For this review, take the finished solid that the model builds, in its own axes (mm). A direction names the side the tool comes from. Round coordinates to 2 decimals unless told otherwise and drop trailing zeros. Write each loop counter-clockwise with the first axis right and the second up, starting at its lowest first coordinate (ties: lowest second). Pieces come first, ordered by that corner, then holes. Notation, with made-up numbers: (-24.5, 69) -> (-19.5, 69) arc R30 cw to (-19.5, 101) -> close; hole circle Ø3 at (1.5, 21). An arc over 180 degrees is marked (long way). Answer in a Markdown table with one row per item. Add a question column.
```python
from build123d import *

# Parameters (mm, degrees)
SKETCH1_W                 = 322.453
SKETCH1_H                 = 14.859
BOSS_EXTRUDE1_DEPTH       = 9.398
SKETCH2_W                 = 6.35
SKETCH2_H                 = 13.335
CUT_EXTRUDE1_DEPTH        = 323.762823192
F_5_CLEARANCE_HOLE1_D     = 3.556
F_5_CLEARANCE_HOLE1_DEPTH = 1.524
F_5_CLEARANCE_HOLE2_D     = 3.556
F_5_CLEARANCE_HOLE2_DEPTH = 14.859
F_5_CLEARANCE_HOLE3_D     = 3.556
FILLET1_R                 = 0.635


with BuildPart() as part:
    # Sketch1 → Boss-Extrude1 (new body)
    with BuildSketch(Plane(origin=(-4.699, 0, 0), x_dir=(0, -1, 0), z_dir=(-1, 0, 0))):
        with Locations((-161.2265, -5.9055)):
            Rectangle(SKETCH1_W, SKETCH1_H)
    extrude(amount=-BOSS_EXTRUDE1_DEPTH)

    # Sketch2 → Cut-Extrude1 (cut, through all)
    with BuildSketch(Plane.XZ):
        with Locations((0, -6.6675)):
            Rectangle(SKETCH2_W, SKETCH2_H)
    extrude(amount=-CUT_EXTRUDE1_DEPTH, mode=Mode.SUBTRACT)

    # #5 Clearance Hole1
    with Locations(Plane(origin=(4.699, 0, 0), x_dir=(0, 0, -1), z_dir=(1, 0, 0))):
        with Locations((8.5725, 307.9115), (8.5725, 317.6905), (8.5725, 298.1325), (8.5725, 288.3535), (8.5725, 278.5745), (8.5725, 268.7955), (8.5725, 259.0165), (8.5725, 249.2375), (8.5725, 239.4585), (8.5725, 229.6795), (8.5725, 219.9005), (8.5725, 210.1215), (8.5725, 200.3425), (8.5725, 190.5635), (8.5725, 180.7845), (8.5725, 171.0055), (8.5725, 161.2265), (8.5725, 151.4475), (8.5725, 141.6685), (8.5725, 131.8895), (8.5725, 122.1105), (8.5725, 112.3315), (8.5725, 102.5525), (8.5725, 92.7735), (8.5725, 82.9945), (8.5725, 73.2155), (8.5725, 63.4365), (8.5725, 53.6575), (8.5725, 43.8785), (8.5725, 34.0995), (8.5725, 24.3205), (8.5725, 14.5415), (8.5725, 4.7625)):
            Hole(F_5_CLEARANCE_HOLE1_D / 2, depth=F_5_CLEARANCE_HOLE1_DEPTH)

    # #5 Clearance Hole2
    with Locations(Plane.XY.offset(1.524)):
        with Locations((0, 307.9115), (0, 317.6905), (0, 298.1325), (0, 288.3535), (0, 278.5745), (0, 268.7955), (0, 259.0165), (0, 249.2375), (0, 239.4585), (0, 229.6795), (0, 219.9005), (0, 210.1215), (0, 200.3425), (0, 190.5635), (0, 180.7845), (0, 171.0055), (0, 161.2265), (0, 151.4475), (0, 141.6685), (0, 131.8895), (0, 122.1105), (0, 112.3315), (0, 102.5525), (0, 92.7735), (0, 82.9945), (0, 73.2155), (0, 63.4365), (0, 53.6575), (0, 43.8785), (0, 34.0995), (0, 24.3205), (0, 14.5415), (0, 4.7625)):
            Hole(F_5_CLEARANCE_HOLE2_D / 2, depth=F_5_CLEARANCE_HOLE2_DEPTH)

    # #5 Clearance Hole3 (through all)
    with Locations(Plane(origin=(-3.175, 0, 0), x_dir=(0, 0, -1), z_dir=(1, 0, 0))):
        with Locations((8.5725, 307.9115), (8.5725, 317.6905), (8.5725, 298.1325), (8.5725, 288.3535), (8.5725, 278.5745), (8.5725, 268.7955), (8.5725, 259.0165), (8.5725, 249.2375), (8.5725, 239.4585), (8.5725, 229.6795), (8.5725, 219.9005), (8.5725, 210.1215), (8.5725, 200.3425), (8.5725, 190.5635), (8.5725, 180.7845), (8.5725, 171.0055), (8.5725, 161.2265), (8.5725, 151.4475), (8.5725, 141.6685), (8.5725, 131.8895), (8.5725, 122.1105), (8.5725, 112.3315), (8.5725, 102.5525), (8.5725, 92.7735), (8.5725, 82.9945), (8.5725, 73.2155), (8.5725, 63.4365), (8.5725, 53.6575), (8.5725, 43.8785), (8.5725, 34.0995), (8.5725, 24.3205), (8.5725, 14.5415), (8.5725, 4.7625)):
            Hole(F_5_CLEARANCE_HOLE3_D / 2)

    # Fillet1
    fillet1_edges = [part.edges().sort_by_distance(p)[0] for p in [
        (-3.937, 322.453, -13.335),
        (-3.937, 0, -13.335),
        (3.937, 0, -13.335),
        (3.937, 322.453, -13.335),
    ]]
    fillet(fillet1_edges, radius=FILLET1_R)


solid = part.part
```
1. We need section B-B (x = 0). Count the separate pieces of the cut face and the enclosed holes in it, plus the area to 3 significant figures.
2. Clearance check with a flat-ended pin moving along its axis: pin 1 Ø3 at (x, y) = (0, 34.1) entering from -Z. State where the tip first meets the part, or that it passes through.
3. We need section C-C (y = 293.5). Write out the cut boundary in (x, z) (3 decimals).
4. Tool access review of faces 1 (the flat face through (-3.175, 159, -7)), 2 (the flat face through (-4, 0, -4)): name each direction out of +Z, -Z, +X, -X, +Y, -Y from which nothing blocks a thin tool from reaching the whole face with its end or side.
5. We need section A-A (z = -4.25). Write out the cut boundary in (x, y) (3 decimals).
6. For L1, parallel to X at y = 136, z = -10.25 (3 decimals); L2, parallel to Z at x = -1.75, y = 256.5, list the stretches that pass through material, from the lowest coordinate up. Write a range as [from, to].
Response:
| question | item | result |
|---|---|---|
| 1 | separate pieces | 34 |
| 1 | enclosed holes | 0 |
| 1 | area | 313 mm2 |
| 2 | pin 1 | through |
| 3 | outline | (-4.699, -13.335) -> (-3.175, -13.335) -> (-3.175, 0) -> (3.175, 0) -> (3.175, -13.335) -> (4.699, -13.335) -> (4.699, 1.524) -> (-4.699, 1.524) -> close |
| 4 | face 1 | -Z, +Y, -Y |
| 4 | face 2 | +Z, -Z, +X, -X, -Y |
| 5 | outline | (-4.699, 0) -> (-3.175, 0) -> (-3.175, 322.453) -> (-4.699, 322.453) -> close; (3.175, 0) -> (4.699, 0) -> (4.699, 322.453) -> (3.175, 322.453) -> close |
| 6 | L1 | [-4.699, -3.175], [3.175, 4.699] |
| 6 | L2 | [0, 1.52] |
